Job drawing, mm, ordinate dimensions from the low corner. One solid piece. Coordinates: 2 decimals unless noted, no trailing zeros. Loops run counter-clockwise (first coordinate to the right, second up) from the corner with the lowest first, then second, coordinate; pieces in that order, holes last. Notation, with made-up numbers: (42, -16.75) - (62, -16.75) arc R23 ccw to (62, 9.25) - close; hole circle Ø1 at (45.5, -30.5). An arc over 180 degrees is marked (long way). One line per question, with ' | ' between items. Start each with the question number.
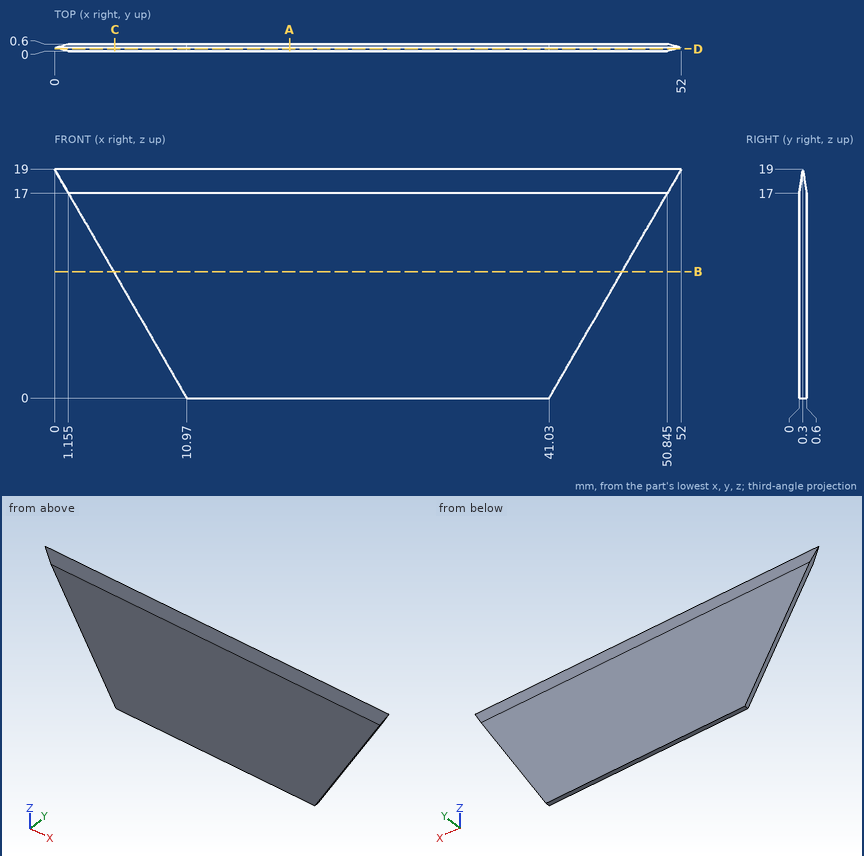
1) Band-saw the part on B-B on z = 10.5. List the corners of the cut face in (x, y).
2) Wall check: line 1 along X through (y, z) = (0.55, 10.75); line 2 along X through (y, z) = (0.3, 6) (1 decimal); line 3 along Y through (x, z) = (24.5, 17.5) (1 decimal). Give the ranges that are in metal, low to high. Write a range as [from, to].
3) Band-saw the part on A-A on x = 19.5. List the corners of the cut face in (y, z).
4) Band-saw the part on D-D on y = 0.2. List the corners of the cut face in (x, z) (1 decimal), then the cut area to 3 significant figures.
5) Band-saw the part on C-C on x = 5. List the corners of the cut face in (y, z).
Values found:
1) outline: (4.91, 0) - (47.09, 0) - (47.09, 0.6) - (4.91, 0.6) - close
2) line 1: [4.76, 47.24] | line 2: [7.5, 44.5] | line 3: [0.1, 0.5]
3) outline: (0, 0) - (0.6, 0) - (0.6, 17) - (0.3, 19) - (0, 17) - close
4) outline: (0.4, 18.3) - (11, 0) - (41, 0) - (51.6, 18.3) - close | area: 745 mm²
5) outline: (0, 10.34) - (0.6, 10.34) - (0.6, 17) - (0.3, 19) - (0, 17) - close
